from build123d import *

# Parameters (mm, degrees)
SKETCH1_R           = 3.05
SKETCH1_R_2         = 2.85
BOSS_EXTRUDE1_DEPTH = 22.5
THREAD1_PITCH       = 0.79375
CUT_EXTRUDE1_REACH  = 73.638
SKETCH12_R          = 2.85
SKETCH13_W          = 4.3
SKETCH13_H          = 8.396908484
BOSS_EXTRUDE2_DEPTH = 22.5
CUT_EXTRUDE2_REACH  = 53.493
SKETCH14_W          = 19.5
SKETCH14_H          = 2.3
FILLET1_R           = 1
FILLET2_R           = 0.5


with BuildPart() as part:
    # Sketch1 → Boss-Extrude1 (new body)
    with BuildSketch(Plane(origin=(0, 0, 0), x_dir=(0, 0, -1), z_dir=(1, 0, 0))):
        with Locations(Location((0, 0, 0), (0, 0, 180))):
            Circle(SKETCH1_R)
        with Locations(Location((0, 0, 0), (0, 0, 180))):
            Circle(SKETCH1_R_2, mode=Mode.SUBTRACT)
    extrude(amount=BOSS_EXTRUDE1_DEPTH)

    # Sweep1: sweep along a path in Sketch4
    with BuildLine(Plane(origin=(0, -2.85, 0), x_dir=(-1, 0, 0), z_dir=(0, -1, 0))) as sweep1_path:
        Line((0, 0), (-22.5, 0))
    # Sketch3 → Sweep1 (sweep)
    with BuildSketch(Plane(origin=(0, 0, 0), x_dir=(0, 0, -1), z_dir=(1, 0, 0))):
        Polygon((-3.05, 0), (3.05, 0), (1.163985807, -17.9442264), (1.163985807, -67.9442264), (-1.136014193, -67.9442264), (-1.136014193, -18.210358526), align=None)
    sweep(path=sweep1_path.line)

    # Sketch7 → CSK for #6 Flat Head Machine Screw (100)1 (revolve, cut)
    with BuildSketch(Plane(origin=(11.25, -62.1942264, -1.163985807), x_dir=(0, 1, 0), z_dir=(1, 0, 0))):
        Polygon((0, 0), (0, 2.3), (1.89865, 2.3), (1.89865, 1.380025208), (3.5433, 0), align=None)
    revolve(axis=Axis((11.25, -62.1942264, -7.513985807), (0, 0, 1)), mode=Mode.SUBTRACT)

    # Thread1: the profile of Thread Profile1 profile screwed along a right-hand helix of 1.159023 turns, 8 arcs to a turn; built about Z, then put on its axis
    thread1_z = Axis((0, 0, 0), (0, 0, 1))
    thread1_corners = [(1.89835, 0, -0.000173205), (2.328279788, 0, 0.248046874), (2.328279788, 0, 0.347265624), (1.89835, 0, 0.595485703)]
    with BuildLine(mode=Mode.PRIVATE) as thread1_profile:
        Line(thread1_corners[0], thread1_corners[1])
        Line(thread1_corners[1], thread1_corners[2])
        Line(thread1_corners[2], thread1_corners[3])
        Line(thread1_corners[3], thread1_corners[0])
    thread1_cap = Face(thread1_profile.wire())
    thread1_turn_angles = [0, 22.5, 45, 67.5, 90, 112.5, 135, 157.5, 180, 202.5, 225, 247.5, 270, 292.5, 315, 337.5, 360]
    thread1_turn_weights = [1, 0.9238795325112867, 1, 0.9238795325112867, 1, 0.9238795325112867, 1, 0.9238795325112867, 1, 0.9238795325112867, 1, 0.9238795325112867, 1, 0.9238795325112867, 1, 0.9238795325112867, 1]
    thread1_turn_rails = [Edge.make_bspline([Vector(p[0], p[1], 0).rotate(thread1_z, thread1_turn_angles[k]) / thread1_turn_weights[k] + Vector(0, 0, p[2] + THREAD1_PITCH * thread1_turn_angles[k] / 360) for k in range(17)], [0, 0, 0, 1, 1, 2, 2, 3, 3, 4, 4, 5, 5, 6, 6, 7, 7, 8, 8, 8], 2, thread1_turn_weights) for p in thread1_corners]
    thread1_turn_sides = [Face.make_surface_from_curves(thread1_turn_rails[p[0]], thread1_turn_rails[p[1]]) for p in [(0, 1), (1, 2), (2, 3), (3, 0)]]
    thread1_last_angles = [360, 382.5, 405, 411.124204706, 417.248409411]
    thread1_last_weights = [1, 0.9238795325112867, 1, 0.9942929639578036, 1]
    thread1_last_rails = [Edge.make_bspline([Vector(p[0], p[1], 0).rotate(thread1_z, thread1_last_angles[k]) / thread1_last_weights[k] + Vector(0, 0, p[2] + THREAD1_PITCH * thread1_last_angles[k] / 360) for k in range(5)], [0, 0, 0, 1, 1, 2, 2, 2], 2, thread1_last_weights) for p in thread1_corners]
    thread1_last_sides = [Face.make_surface_from_curves(thread1_last_rails[p[0]], thread1_last_rails[p[1]]) for p in [(0, 1), (1, 2), (2, 3), (3, 0)]]
    thread1 = Plane(origin=(11.25, -62.1942264, 0.216039402), x_dir=(1, 0, 0), z_dir=(0, 0, 1)) * Solid(Shell([*thread1_turn_sides, *thread1_last_sides, thread1_cap, thread1_cap.rotate(thread1_z, 417.248409411).moved(Location((0, 0, THREAD1_PITCH * 417.248409411 / 360)))]))
    add(thread1, mode=Mode.SUBTRACT)

    # Sketch12 → Cut-Extrude1 (cut, up to next)
    with BuildSketch(Plane(origin=(22.5, 0, 0), x_dir=(0, 0, -1), z_dir=(1, 0, 0)), mode=Mode.PRIVATE) as cut_extrude1_sk1:
        with Locations(Location((0, 0, 0), (0, 0, 180))):
            Circle(SKETCH12_R)
    cut_extrude1_tool1 = extrude(cut_extrude1_sk1.sketch, amount=-CUT_EXTRUDE1_REACH, mode=Mode.PRIVATE) & part.part
    add(cut_extrude1_tool1.solids().sort_by_distance((22.5, 0, 0))[0], mode=Mode.SUBTRACT)

    # Sketch13 → Boss-Extrude2 (add)
    with BuildSketch(Plane(origin=(22.5, 0, 0), x_dir=(0, 0, -1), z_dir=(1, 0, 0))):
        with Locations((3.313985807, -38.745772158)):
            Rectangle(SKETCH13_W, SKETCH13_H)
    extrude(amount=-BOSS_EXTRUDE2_DEPTH)

    # Sketch14 → Cut-Extrude2 (cut, up to next)
    with BuildSketch(Plane.XZ.offset(42.9442264), mode=Mode.PRIVATE) as cut_extrude2_sk1:
        with Locations((11.25, -2.313985807)):
            Rectangle(SKETCH14_W, SKETCH14_H)
    cut_extrude2_tool1 = extrude(cut_extrude2_sk1.sketch, amount=-CUT_EXTRUDE2_REACH, mode=Mode.PRIVATE) & part.part
    add(cut_extrude2_tool1.solids().sort_by_distance((11.25, -42.944226, -2.313986))[0], mode=Mode.SUBTRACT)

    # Fillet1
    fillet1_edges = [part.edges().sort_by_distance(p)[0] for p in [
        (22.5, -67.9442264, -0.013985807),
        (0, -67.9442264, -0.013985807),
    ]]
    fillet(fillet1_edges, radius=FILLET1_R)

    # Fillet2
    fillet2_edges = [part.edges().sort_by_distance(p)[0] for p in [
        (0, -34.547317916, -3.313985807),
        (0, -38.745772158, -5.463985807),
        (11.25, -34.547317916, -5.463985807),
        (0, -42.9442264, -3.313985807),
        (11.25, -42.9442264, -5.463985807),
        (22.5, -42.9442264, -3.313985807),
        (22.5, -38.745772158, -5.463985807),
        (22.5, -34.547317916, -3.313985807),
        (1.5, -42.9442264, -2.313985807),
        (11.25, -42.9442264, -3.463985807),
        (21, -42.9442264, -2.313985807),
        (11.25, -34.547317916, -3.463985807),
        (21, -34.547317916, -2.313985807),
        (1.5, -34.547317916, -2.313985807),
    ]]
    fillet(fillet2_edges, radius=FILLET2_R)


solid = part.part
Here's how the part is built. I have some questions about the finished solid (model axes, mm). A direction names the side the tool comes from. Round coordinates to 2 decimals unless told otherwise and drop trailing zeros. Loops run counter-clockwise (first coordinate to the right, second up) from the corner with the lowest first, then second, coordinate; pieces in that order, holes last. Notation, with made-up numbers: M 48,80 L 58,80 A13 cw 58,89 Z; hole C -19.5,49.25 d5. An arc over 180 degrees is marked long. Write each question's results on one line, items separated by ' | '. Start each with the question number.
(1) Will these pins go through, and if not, where does the flat tip stop? P1, Ø1.1, axis at x = 9.5, z = -3, coming from the +Y side; P2, Ø4, axis at x = 15, z = -2.5, coming from the +Y side; P3, Ø2, axis at x = 13, y = -38.5, coming from the +Z side.
(2) I want a section at A-A (x = 20.25). Please give me the cut outline in (y, z), then the cut area to 3 significant figures.
(3) I want a section at D-D (y = -26). Please give me the cut outline in (x, z), then the cut area to 4 significant figures.
(4) Thinking about a two-plate mould opening in Y: for faces 4 (the flat face through (11, -67.944, 0)), 5 (the cylindrical face through (11.09, 2.78, -0.62)), 6 (the flat face through (11, -39, -5.464)), which applies, pulls with the +Y half, pulls with the -Y half, needs draft (parallel to the pull), parting line crosses it, or undercut?
(5) If I drill on probe 1 along Z at (x, y) = (17.25, -39); probe 2 along Y at (x, z) = (17.5, 0); probe 3 along Y at (x, z) = (11.25, 0.5), over which ranges is the centre line in solid material (lowest first)? Write a range as from..to.
(6) On a 3-axis mill with a long thin cutter (end or side, diameter ignored), from which of +Z, -Z, +X, -X, +Y, -Y can I reach the whole of each face in a straight line? I mean faces 1 (the flat face through (21, -39, -2)), 2 (the flat face through (11.41, -9.41, -2.06)), 3 (the flat face through (11, -39, -3.464)). Say none if no direction works.
(7) I want a section at B-B (y = 0). Please give me the cut outline in (x, z).
(8) I want a section at C-C (z = 2.25). Please give me the cut outline in (x, y).
Solved:
1) P1: stops at y = 1.82 | P2: stops at y = 3.01 | P3: stops at z = 1.14
2) outline: M -67.94,-1.16 L -17.94,-1.16 L -0.63,-2.98 A3.05 ccw long -0.63,2.98 L -18.21,1.14 L -67.94,1.14 Z; M -42.94,-4.96 A0.5 ccw -42.44,-5.46 L -35.05,-5.46 A0.5 ccw -34.55,-4.96 L -34.55,-3.96 A0.5 ccw -35.05,-3.46 L -42.44,-3.46 A0.5 ccw -42.94,-3.96 Z; hole C 0,0 d5.7 | area: 196 mm²
3) outline: M 0,-1.16 L 22.5,-1.16 L 22.5,1.14 L 0,1.14 Z | area: 51.75 mm²
4) face 4: pulls with the -Y half | face 5: undercut | face 6: needs draft
5) probe 1: z = -5.46..-3.46, -1.16..1.14 | probe 2: y = -67.94..-2.85, 2.85..3.05 | probe 3: y = -67.94..-64.09, -60.15..-2.81, 2.81..3.01
6) face 1: -Y | face 2: -Z, +X, -X | face 3: +Y, -Y
7) outline: M 0,-3.05 L 22.5,-3.05 L 22.5,-2.85 L 0,-2.85 Z; M 0,2.85 L 22.5,2.85 L 22.5,3.05 L 0,3.05 Z
8) outline: M 0,-7.61 L 22.5,-7.61 L 22.5,-1.75 L 0,-1.75 Z; M 0,1.75 L 22.5,1.75 L 22.5,2.06 L 0,2.06 Z
